Check sheet for the modelled part. Datum: model origin and axes. Units: mm. Face numbers are marked on the shaded views. A direction names the side the tool comes from. Round coordinates to 2 decimals unless told otherwise and drop trailing zeros. Write each loop counter-clockwise with the first axis right and the second up, starting at its lowest first coordinate (ties: lowest second). Pieces come first, ordered by that corner, then holes. Notation, with made-up numbers: M 61.25,-10 L 76.25,-10 A17 ccw 76.25,2 Z; hole C 58,39 d1. An arc over 180 degrees is marked long. Put each result on its own line as item: value.
```python
from build123d import *

# Parameters (mm, degrees)
SKETCH1_R               = 10
BOSS_EXTRUDE1_DEPTH     = 40
CUT_EXTRUDE1_DEPTH      = 20
CUT_EXTRUDE1_DEPTH_BACK = 40
SKETCH2_W               = 20
SKETCH2_H               = 28.944782362
SKETCH3_R               = 5
CUT_EXTRUDE3_DEPTH      = 40


with BuildPart() as part:
    # Sketch1 → Boss-Extrude1 (new body)
    with BuildSketch(Plane.XY):
        Circle(SKETCH1_R)
        with BuildLine():
            Line((53.512258846, 10), (0, 10))
            ThreePointArc((0, 10), (7.071067812, 7.071067812), (10, 0))
            ThreePointArc((10, 0), (7.071067812, -7.071067812), (0, -10))
            Line((0, -10), (53.512258846, -10))
            Line((53.512258846, -10), (53.512258846, 10))
        make_face()
    extrude(amount=BOSS_EXTRUDE1_DEPTH)

    # Sketch2 → Cut-Extrude1 (cut, two sides: drawn at the far end of the back side and taken through both)
    with BuildSketch(Plane(origin=(0, 0, 0), x_dir=(0, 0, -1), z_dir=(1, 0, 0)).offset(-CUT_EXTRUDE1_DEPTH_BACK)):
        with Locations((-20, 0)):
            Rectangle(SKETCH2_W, SKETCH2_H)
    extrude(amount=CUT_EXTRUDE1_DEPTH + CUT_EXTRUDE1_DEPTH_BACK, mode=Mode.SUBTRACT)

    # Sketch3 → Cut-Extrude3 (cut)
    with BuildSketch(Plane.XY.offset(40)):
        Circle(SKETCH3_R)
    extrude(amount=-CUT_EXTRUDE3_DEPTH, mode=Mode.SUBTRACT)


solid = part.part
```
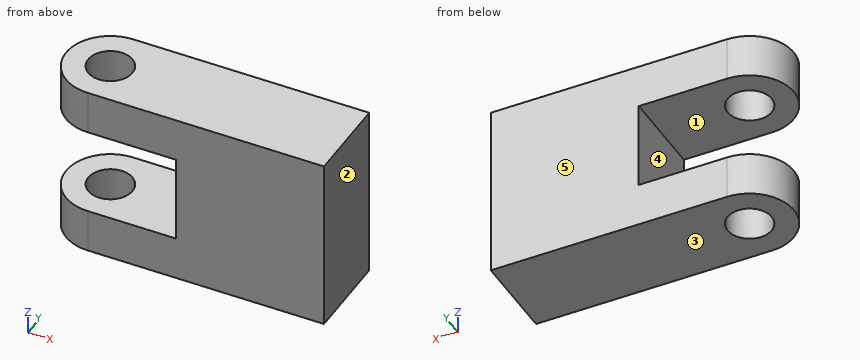
1. Depth check by flat-ended pin: pin 1 Ø1 at (y, z) = (-5.5, 6) entering from -X. Enter the tip coordinate at first touch or a pass-through.
Computed values:
pin 1: stops at x = -8.66
2. Cross-section at A-A (y = 0). Enter the section's corners in (x, z), then the cut area to 3 significant figures.
Computed values:
outline: M -10,0 L -5,0 L -5,10 L -10,10 Z; M -10,30 L -5,30 L -5,40 L -10,40 Z; M 5,0 L 53.51,0 L 53.51,40 L 5,40 L 5,30 L 20,30 L 20,10 L 5,10 Z
area: 1,740 mm2
3. Cross-section at C-C (y = 3.25). Enter the section's corners in (x, z).
Computed values:
outline: M -9.46,0 L -3.8,0 L -3.8,10 L -9.46,10 Z; M -9.46,30 L -3.8,30 L -3.8,40 L -9.46,40 Z; M 3.8,0 L 53.51,0 L 53.51,40 L 3.8,40 L 3.8,30 L 20,30 L 20,10 L 3.8,10 Z
4. Access from +Z, -Z, +X, -X, +Y, -Y to the whole of each face (thin tool, end or side, straight path). Record for the marked faces 4 and 5.
Computed values:
face 4: -X, +Y, -Y
face 5: +Z, -Z, +X, -X, +Y
5. Cross-section at D-D (z = 20). Enter the section's corners in (x, y), then the cut area to 3 significant figures.
Computed values:
outline: M 20,-10 L 53.51,-10 L 53.51,10 L 20,10 Z
area: 670 mm2
6. Scan lines: probe 1 along Z at (x, y) = (-7, 3); probe 2 along Y at (x, z) = (0, 4); probe 3 along X at (y, z) = (5.5, 17). Record each from-to range of solid material in increasing order.
Computed values:
probe 1: z = 0 to 10, 30 to 40
probe 2: y = -10 to -5, 5 to 10
probe 3: x = 20 to 53.51
7. Cross-section at B-B (z = 7). Enter the section's corners in (x, y), then the cut area to 3 significant figures.
Computed values:
outline: M 0,-10 L 53.51,-10 L 53.51,10 L 0,10 A10 ccw Z; hole C 0,0 d10
area: 1,150 mm2
8. Release check for a two-part mould opening along Z. For the marked faces 1, 2 and 3 record: +Z half, -Z half, draft (parallel to the pull), parting line (faces both ways), or undercut.
Computed values:
face 1: undercut
face 2: draft
face 3: -Z half
